Autodesk Fusion 360 part; units mm, degrees
sketch "Sketch1" plane through (0, 0, 0) normal (0, 0, 1) x (1, 0, 0)
  circle A0 centre (0, 0) radius 3.35 construction
  line L0 (1.282, 3.095) -> (-1.282, 3.095)
  line L1 (-1.282, 3.095) -> (-3.095, 1.282)
  line L2 (-3.095, 1.282) -> (-3.095, -1.282)
  line L3 (-3.095, -1.282) -> (-1.282, -3.095)
  line L4 (-1.282, -3.095) -> (1.282, -3.095)
  line L5 (1.282, -3.095) -> (3.095, -1.282)
  line L6 (3.095, -1.282) -> (3.095, 1.282)
  line L7 (3.095, 1.282) -> (1.282, 3.095)
  dimension "d1" = 6.7
extrude "Extrude1" add sketch "Sketch1" along normal blind 7
chamfer "Chamfer1" distance 0.5 angle 45 8 edges at (-2.1885, 2.1885, 7) (-3.095, 0, 7) (-2.1885, -2.1885, 7) (2.1885, -2.1885, 7) (3.095, 0, 7) (2.1885, 2.1885, 7) (0, 3.095, 7) (0, -3.095, 7)
chamfer "Chamfer2" distance 0.5 angle 45 8 edges at (2.1885, -2.1885, 0) (-2.1885, -2.1885, 0) (-3.095, 0, 0) (-2.1885, 2.1885, 0) (0, 3.095, 0) (2.1885, 2.1885, 0) (3.095, 0, 0) (0, -3.095, 0)
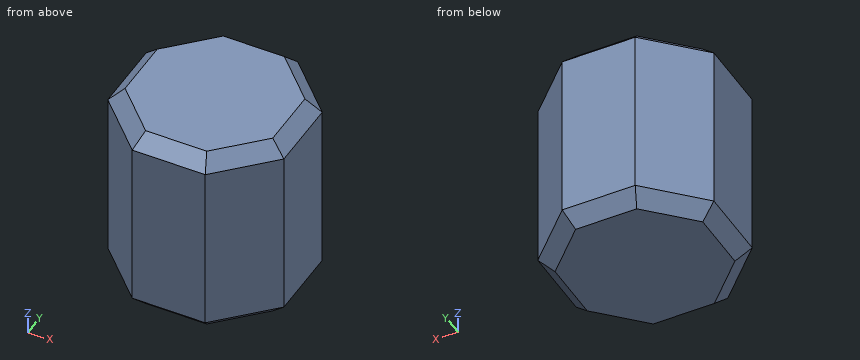
Geometry check sheet. Reference: the model listing, model coordinates, mm. Round coordinates to 2 decimals unless told otherwise and drop trailing zeros. Loops run counter-clockwise (first coordinate to the right, second up) from the corner with the lowest first, then second, coordinate; pieces in that order, holes last.
Item 1: Cross-section at B-B on y = -1.75. Record the boundary of the cut face in (x, z).
Item 2: Cross-section at A-A on z = 6. Record the boundary of the cut face in (x, y) (3 decimals).
Item 3: Thickness scan on line 1 (X direction, y = 2, z = 4.25); line 2 (X direction, y = 2.25, z = 2.5). Record the ranges inside material, lowest first.
Answer sheet:
1. outline: (-2.63, 0.5) - (-1.92, 0) - (1.92, 0) - (2.63, 0.5) - (2.63, 6.5) - (1.92, 7) - (-1.92, 7) - (-2.63, 6.5) - close
2. outline: (-3.095, -1.282) - (-1.282, -3.095) - (1.282, -3.095) - (3.095, -1.282) - (3.095, 1.282) - (1.282, 3.095) - (-1.282, 3.095) - (-3.095, 1.282) - close
3. line 1: x = -2.38 to 2.38
3. line 2: x = -2.13 to 2.13
